Geometry check sheet. Reference: the model listing, model coordinates, mm. Give positions to 0.01 mm unless a question says otherwise; leave off trailing zeros. Loops run counter-clockwise (first coordinate to the right, second up) from the corner with the lowest first, then second, coordinate; pieces in that order, holes last. Notation, with made-up numbers: (59, 75) -> (76, 75) arc R38 ccw to (76, 114) -> close; hole circle Ø11 at (-21, -0.75). An arc over 180 degrees is marked (long way). Write each question's results on one line, items separated by ' | '. Start each with the question number.
1) Sectioned sample at B-B on z = 52. Record the cut outline in (x, y).
2) Sectioned sample at C-C on y = 7.75. Count the separate pieces of the cut face and the enclosed holes in it, then the cut area to 3 significant figures.
3) Scan lines: line 1 (Z direction, x = 24, y = 2.75); line 2 (X direction, y = 3.25, z = -28); line 3 (Z direction, x = -26, y = 5). Record each from-to range of solid material in increasing order. Write a range as from..to.
4) Depth check by flat-ended pin: pin 1 (5.5 mm diameter, centred on x = 24, z = 27.5, fed in from +Y). Enter the tip coordinate at first touch or a pass-through.
5) Sectioned sample at A-A on x = 24. Record the cut outline in (y, z), then the cut area to 3 significant figures.
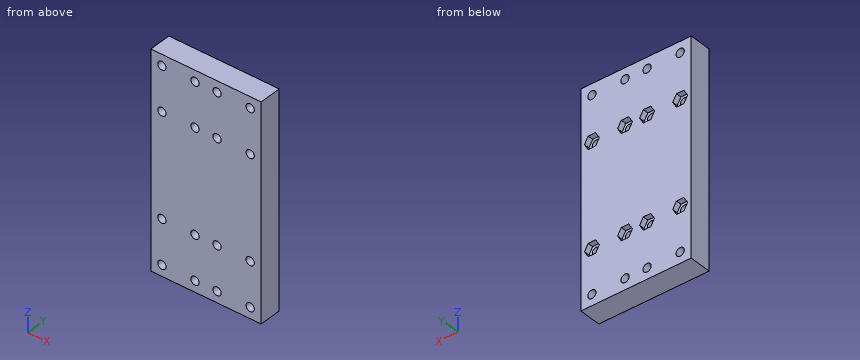
```python
from build123d import *

# Parameters (mm, degrees)
SKETCH1_W                      = 60
SKETCH1_H                      = 116
BOSS_EXTRUDE1_DEPTH            = 12
CUT_EXTRUDE1_REACH             = 14
SKETCH2_R                      = 2.25
CUT_EXTRUDE1_DIRECTION_2_DEPTH = 1
CUT_EXTRUDE2_DEPTH             = 1
CUT_EXTRUDE2_DEPTH_BACK        = 3


with BuildPart() as part:
    # Sketch1 → Boss-Extrude1 (new body)
    with BuildSketch(Plane(origin=(0, 0, 0), x_dir=(1, 0, 0), z_dir=(0, 1, 0))):
        Rectangle(SKETCH1_W, SKETCH1_H)
    extrude(amount=BOSS_EXTRUDE1_DEPTH)

    # Sketch2 → Cut-Extrude1 (cut, up to next)
    with BuildSketch(Plane(origin=(0, 12, 0), x_dir=(1, 0, 0), z_dir=(0, 1, 0)), mode=Mode.PRIVATE) as cut_extrude1_sk1:
        with Locations((-24, 52)):
            Circle(SKETCH2_R)
    cut_extrude1_tool1 = extrude(cut_extrude1_sk1.sketch, amount=-CUT_EXTRUDE1_REACH, mode=Mode.PRIVATE) & part.part
    add(cut_extrude1_tool1.solids().sort_by_distance((-24, 12, -52))[0], mode=Mode.SUBTRACT)
    # Sketch2 → Cut-Extrude1 (cut, up to next)
    with BuildSketch(Plane(origin=(0, 12, 0), x_dir=(1, 0, 0), z_dir=(0, 1, 0)), mode=Mode.PRIVATE) as cut_extrude1_sk2:
        with Locations((-6, 52)):
            Circle(SKETCH2_R)
    cut_extrude1_tool2 = extrude(cut_extrude1_sk2.sketch, amount=-CUT_EXTRUDE1_REACH, mode=Mode.PRIVATE) & part.part
    add(cut_extrude1_tool2.solids().sort_by_distance((-6, 12, -52))[0], mode=Mode.SUBTRACT)
    # Sketch2 → Cut-Extrude1 (cut, up to next)
    with BuildSketch(Plane(origin=(0, 12, 0), x_dir=(1, 0, 0), z_dir=(0, 1, 0)), mode=Mode.PRIVATE) as cut_extrude1_sk3:
        with Locations((-24, 28)):
            Circle(SKETCH2_R)
    cut_extrude1_tool3 = extrude(cut_extrude1_sk3.sketch, amount=-CUT_EXTRUDE1_REACH, mode=Mode.PRIVATE) & part.part
    add(cut_extrude1_tool3.solids().sort_by_distance((-24, 12, -28))[0], mode=Mode.SUBTRACT)
    # Sketch2 → Cut-Extrude1 (cut, up to next)
    with BuildSketch(Plane(origin=(0, 12, 0), x_dir=(1, 0, 0), z_dir=(0, 1, 0)), mode=Mode.PRIVATE) as cut_extrude1_sk4:
        with Locations((-6, 28)):
            Circle(SKETCH2_R)
    cut_extrude1_tool4 = extrude(cut_extrude1_sk4.sketch, amount=-CUT_EXTRUDE1_REACH, mode=Mode.PRIVATE) & part.part
    add(cut_extrude1_tool4.solids().sort_by_distance((-6, 12, -28))[0], mode=Mode.SUBTRACT)
    # Sketch2 → Cut-Extrude1 (cut, up to next)
    with BuildSketch(Plane(origin=(0, 12, 0), x_dir=(1, 0, 0), z_dir=(0, 1, 0)), mode=Mode.PRIVATE) as cut_extrude1_sk5:
        with Locations((6, 28)):
            Circle(SKETCH2_R)
    cut_extrude1_tool5 = extrude(cut_extrude1_sk5.sketch, amount=-CUT_EXTRUDE1_REACH, mode=Mode.PRIVATE) & part.part
    add(cut_extrude1_tool5.solids().sort_by_distance((6, 12, -28))[0], mode=Mode.SUBTRACT)
    # Sketch2 → Cut-Extrude1 (cut, up to next)
    with BuildSketch(Plane(origin=(0, 12, 0), x_dir=(1, 0, 0), z_dir=(0, 1, 0)), mode=Mode.PRIVATE) as cut_extrude1_sk6:
        with Locations((24, 28)):
            Circle(SKETCH2_R)
    cut_extrude1_tool6 = extrude(cut_extrude1_sk6.sketch, amount=-CUT_EXTRUDE1_REACH, mode=Mode.PRIVATE) & part.part
    add(cut_extrude1_tool6.solids().sort_by_distance((24, 12, -28))[0], mode=Mode.SUBTRACT)
    # Sketch2 → Cut-Extrude1 (cut, up to next)
    with BuildSketch(Plane(origin=(0, 12, 0), x_dir=(1, 0, 0), z_dir=(0, 1, 0)), mode=Mode.PRIVATE) as cut_extrude1_sk7:
        with Locations((6, 52)):
            Circle(SKETCH2_R)
    cut_extrude1_tool7 = extrude(cut_extrude1_sk7.sketch, amount=-CUT_EXTRUDE1_REACH, mode=Mode.PRIVATE) & part.part
    add(cut_extrude1_tool7.solids().sort_by_distance((6, 12, -52))[0], mode=Mode.SUBTRACT)
    # Sketch2 → Cut-Extrude1 (cut, up to next)
    with BuildSketch(Plane(origin=(0, 12, 0), x_dir=(1, 0, 0), z_dir=(0, 1, 0)), mode=Mode.PRIVATE) as cut_extrude1_sk8:
        with Locations((24, 52)):
            Circle(SKETCH2_R)
    cut_extrude1_tool8 = extrude(cut_extrude1_sk8.sketch, amount=-CUT_EXTRUDE1_REACH, mode=Mode.PRIVATE) & part.part
    add(cut_extrude1_tool8.solids().sort_by_distance((24, 12, -52))[0], mode=Mode.SUBTRACT)
    # Sketch2 → Cut-Extrude1 (cut, up to next)
    with BuildSketch(Plane(origin=(0, 12, 0), x_dir=(1, 0, 0), z_dir=(0, 1, 0)), mode=Mode.PRIVATE) as cut_extrude1_sk9:
        with Locations((24, -52)):
            Circle(SKETCH2_R)
    cut_extrude1_tool9 = extrude(cut_extrude1_sk9.sketch, amount=-CUT_EXTRUDE1_REACH, mode=Mode.PRIVATE) & part.part
    add(cut_extrude1_tool9.solids().sort_by_distance((24, 12, 52))[0], mode=Mode.SUBTRACT)
    # Sketch2 → Cut-Extrude1 (cut, up to next)
    with BuildSketch(Plane(origin=(0, 12, 0), x_dir=(1, 0, 0), z_dir=(0, 1, 0)), mode=Mode.PRIVATE) as cut_extrude1_sk10:
        with Locations((6, -52)):
            Circle(SKETCH2_R)
    cut_extrude1_tool10 = extrude(cut_extrude1_sk10.sketch, amount=-CUT_EXTRUDE1_REACH, mode=Mode.PRIVATE) & part.part
    add(cut_extrude1_tool10.solids().sort_by_distance((6, 12, 52))[0], mode=Mode.SUBTRACT)
    # Sketch2 → Cut-Extrude1 (cut, up to next)
    with BuildSketch(Plane(origin=(0, 12, 0), x_dir=(1, 0, 0), z_dir=(0, 1, 0)), mode=Mode.PRIVATE) as cut_extrude1_sk11:
        with Locations((24, -28)):
            Circle(SKETCH2_R)
    cut_extrude1_tool11 = extrude(cut_extrude1_sk11.sketch, amount=-CUT_EXTRUDE1_REACH, mode=Mode.PRIVATE) & part.part
    add(cut_extrude1_tool11.solids().sort_by_distance((24, 12, 28))[0], mode=Mode.SUBTRACT)
    # Sketch2 → Cut-Extrude1 (cut, up to next)
    with BuildSketch(Plane(origin=(0, 12, 0), x_dir=(1, 0, 0), z_dir=(0, 1, 0)), mode=Mode.PRIVATE) as cut_extrude1_sk12:
        with Locations((6, -28)):
            Circle(SKETCH2_R)
    cut_extrude1_tool12 = extrude(cut_extrude1_sk12.sketch, amount=-CUT_EXTRUDE1_REACH, mode=Mode.PRIVATE) & part.part
    add(cut_extrude1_tool12.solids().sort_by_distance((6, 12, 28))[0], mode=Mode.SUBTRACT)
    # Sketch2 → Cut-Extrude1 (cut, up to next)
    with BuildSketch(Plane(origin=(0, 12, 0), x_dir=(1, 0, 0), z_dir=(0, 1, 0)), mode=Mode.PRIVATE) as cut_extrude1_sk13:
        with Locations((-6, -28)):
            Circle(SKETCH2_R)
    cut_extrude1_tool13 = extrude(cut_extrude1_sk13.sketch, amount=-CUT_EXTRUDE1_REACH, mode=Mode.PRIVATE) & part.part
    add(cut_extrude1_tool13.solids().sort_by_distance((-6, 12, 28))[0], mode=Mode.SUBTRACT)
    # Sketch2 → Cut-Extrude1 (cut, up to next)
    with BuildSketch(Plane(origin=(0, 12, 0), x_dir=(1, 0, 0), z_dir=(0, 1, 0)), mode=Mode.PRIVATE) as cut_extrude1_sk14:
        with Locations((-24, -28)):
            Circle(SKETCH2_R)
    cut_extrude1_tool14 = extrude(cut_extrude1_sk14.sketch, amount=-CUT_EXTRUDE1_REACH, mode=Mode.PRIVATE) & part.part
    add(cut_extrude1_tool14.solids().sort_by_distance((-24, 12, 28))[0], mode=Mode.SUBTRACT)
    # Sketch2 → Cut-Extrude1 (cut, up to next)
    with BuildSketch(Plane(origin=(0, 12, 0), x_dir=(1, 0, 0), z_dir=(0, 1, 0)), mode=Mode.PRIVATE) as cut_extrude1_sk15:
        with Locations((-6, -52)):
            Circle(SKETCH2_R)
    cut_extrude1_tool15 = extrude(cut_extrude1_sk15.sketch, amount=-CUT_EXTRUDE1_REACH, mode=Mode.PRIVATE) & part.part
    add(cut_extrude1_tool15.solids().sort_by_distance((-6, 12, 52))[0], mode=Mode.SUBTRACT)
    # Sketch2 → Cut-Extrude1 (cut, up to next)
    with BuildSketch(Plane(origin=(0, 12, 0), x_dir=(1, 0, 0), z_dir=(0, 1, 0)), mode=Mode.PRIVATE) as cut_extrude1_sk16:
        with Locations((-24, -52)):
            Circle(SKETCH2_R)
    cut_extrude1_tool16 = extrude(cut_extrude1_sk16.sketch, amount=-CUT_EXTRUDE1_REACH, mode=Mode.PRIVATE) & part.part
    add(cut_extrude1_tool16.solids().sort_by_distance((-24, 12, 52))[0], mode=Mode.SUBTRACT)

    # Sketch2 → Cut-Extrude1 direction 2 (cut)
    with BuildSketch(Plane(origin=(0, 12, 0), x_dir=(1, 0, 0), z_dir=(0, 1, 0))):
        with Locations((-24, 52)):
            Circle(SKETCH2_R)
        with Locations((-6, 52)):
            Circle(SKETCH2_R)
        with Locations((-24, 28)):
            Circle(SKETCH2_R)
        with Locations((-6, 28)):
            Circle(SKETCH2_R)
        with Locations((6, 28)):
            Circle(SKETCH2_R)
        with Locations((24, 28)):
            Circle(SKETCH2_R)
        with Locations((6, 52)):
            Circle(SKETCH2_R)
        with Locations((24, 52)):
            Circle(SKETCH2_R)
        with Locations((24, -52)):
            Circle(SKETCH2_R)
        with Locations((6, -52)):
            Circle(SKETCH2_R)
        with Locations((24, -28)):
            Circle(SKETCH2_R)
        with Locations((6, -28)):
            Circle(SKETCH2_R)
        with Locations((-6, -28)):
            Circle(SKETCH2_R)
        with Locations((-24, -28)):
            Circle(SKETCH2_R)
        with Locations((-6, -52)):
            Circle(SKETCH2_R)
        with Locations((-24, -52)):
            Circle(SKETCH2_R)
    extrude(amount=CUT_EXTRUDE1_DIRECTION_2_DEPTH, mode=Mode.SUBTRACT)

    # Sketch3 → Cut-Extrude2 (cut, two sides)
    with BuildSketch(Plane(origin=(0, 12, 0), x_dir=(1, 0, 0), z_dir=(0, 1, 0))) as cut_extrude2_sk:
        Polygon((-19.958548116, -28), (-21.979274058, -24.5), (-26.020725942, -24.5), (-28.041451884, -28), (-26.020725942, -31.5), (-21.979274058, -31.5), align=None)
        Polygon((-1.958548116, -28), (-3.979274058, -24.5), (-8.020725942, -24.5), (-10.041451884, -28), (-8.020725942, -31.5), (-3.979274058, -31.5), align=None)
        Polygon((3.979274058, -31.5), (1.958548116, -28), (3.979274058, -24.5), (8.020725942, -24.5), (10.041451884, -28), (8.020725942, -31.5), align=None)
        Polygon((21.979274058, -31.5), (19.958548116, -28), (21.979274058, -24.5), (26.020725942, -24.5), (28.041451884, -28), (26.020725942, -31.5), align=None)
        Polygon((26.020725942, 31.5), (21.979274058, 31.5), (19.958548116, 28), (21.979274058, 24.5), (26.020725942, 24.5), (28.041451884, 28), align=None)
        Polygon((8.020725942, 31.5), (3.979274058, 31.5), (1.958548116, 28), (3.979274058, 24.5), (8.020725942, 24.5), (10.041451884, 28), align=None)
        Polygon((-3.979274058, 31.5), (-1.958548116, 28), (-3.979274058, 24.5), (-8.020725942, 24.5), (-10.041451884, 28), (-8.020725942, 31.5), align=None)
        Polygon((-21.979274058, 31.5), (-19.958548116, 28), (-21.979274058, 24.5), (-26.020725942, 24.5), (-28.041451884, 28), (-26.020725942, 31.5), align=None)
    extrude(amount=CUT_EXTRUDE2_DEPTH, mode=Mode.SUBTRACT)
    extrude(cut_extrude2_sk.sketch, amount=-CUT_EXTRUDE2_DEPTH_BACK, mode=Mode.SUBTRACT)


solid = part.part
```
Result:
1) outline: (-30, 0) -> (-26.25, 0) -> (-26.25, 12) -> (-30, 12) -> close; (-21.75, 0) -> (-8.25, 0) -> (-8.25, 12) -> (-21.75, 12) -> close; (-3.75, 0) -> (3.75, 0) -> (3.75, 12) -> (-3.75, 12) -> close; (8.25, 0) -> (21.75, 0) -> (21.75, 12) -> (8.25, 12) -> close; (26.25, 0) -> (30, 0) -> (30, 12) -> (26.25, 12) -> close
2) separate pieces: 1 | enclosed holes: 16 | area: 6,710 mm^2
3) line 1: -58..-54.25, -49.75..-30.25, -25.75..25.75, 30.25..49.75, 54.25..58 | line 2: -30..-26.25, -21.75..-8.25, -3.75..3.75, 8.25..21.75, 26.25..30 | line 3: -58..-53.03, -50.97..-29.03, -26.97..26.97, 29.03..50.97, 53.03..58
4) pin 1: y = 9
5) outline: (0, -58) -> (12, -58) -> (12, -54.25) -> (0, -54.25) -> close; (0, -49.75) -> (12, -49.75) -> (12, -31.5) -> (9, -31.5) -> (9, -30.25) -> (0, -30.25) -> close; (0, -25.75) -> (9, -25.75) -> (9, -24.5) -> (12, -24.5) -> (12, 24.5) -> (9, 24.5) -> (9, 25.75) -> (0, 25.75) -> close; (0, 30.25) -> (9, 30.25) -> (9, 31.5) -> (12, 31.5) -> (12, 49.75) -> (0, 49.75) -> close; (0, 54.25) -> (12, 54.25) -> (12, 58) -> (0, 58) -> close | area: 1,160 mm^2
